from build123d import *

# Parameters (mm, degrees)
EXTRUDE1_DEPTH            = 32.5
SKETCH2_W                 = 70
SKETCH2_H                 = 1.7
CUT_EXTRUDE1_DEPTH        = 124.086646311
M5_CLEARANCE_HOLE1_D      = 5.5
M5X0_8_TAPPED_HOLE1_D     = 4.2
M5X0_8_TAPPED_HOLE1_DEPTH = 19.05
M5X0_8_TAPPED_HOLE1_TIP   = 1.2618073
F_5_0_5_DIAMETER_HOLE1_D  = 5
M8X1_25_TAPPED_HOLE1_D    = 6.8
F_6_0_6_DIAMETER_HOLE1_D  = 6


with BuildPart() as part:
    # Sketch1 → Extrude1 (new, symmetric)
    with BuildSketch(Plane.XY):
        with BuildLine():
            Line((0, 0), (98, 0))
            Line((98, 0), (98, 12.7))
            Line((98, 12.7), (25.4, 12.7))
            ThreePointArc((25.4, 12.7), (16.419743879, 16.419743879), (12.7, 25.4))
            Line((12.7, 25.4), (12.7, 36.35))
            Line((12.7, 36.35), (0, 36.35))
            Line((0, 36.35), (0, 0))
        make_face()
    extrude(amount=EXTRUDE1_DEPTH, both=True)

    # Sketch2 → Cut-Extrude1 (cut, through all)
    with BuildSketch(Plane(origin=(0, 0, -32.5), x_dir=(-1, 0, 0), z_dir=(0, 0, -1))):
        with Locations((-63, 11.85)):
            Rectangle(SKETCH2_W, SKETCH2_H)
    extrude(amount=-CUT_EXTRUDE1_DEPTH, mode=Mode.SUBTRACT)

    # M5 Clearance Hole1 (through all)
    with Locations(Plane.XZ):
        with Locations((53.7, 15), (91.7, 15), (91.7, -15), (53.7, -15)):
            Hole(M5_CLEARANCE_HOLE1_D / 2)

    # M5x0.8 Tapped Hole1
    with Locations(Plane(origin=(0, 36.35, 0), x_dir=(-1, 0, 0), z_dir=(0, 1, 0))):
        with Locations((-6.35, 22.5), (-6.35, -22.5)):
            Hole(M5X0_8_TAPPED_HOLE1_D / 2, depth=M5X0_8_TAPPED_HOLE1_DEPTH)
            with Locations((0, 0, -(M5X0_8_TAPPED_HOLE1_DEPTH + M5X0_8_TAPPED_HOLE1_TIP / 2))):  # 118° drill point
                Cone(0, M5X0_8_TAPPED_HOLE1_D / 2, M5X0_8_TAPPED_HOLE1_TIP, mode=Mode.SUBTRACT)

    # Ø5.0 (5) Diameter Hole1 (through all)
    with Locations(Plane.XZ):
        with Locations((46.70001183, 12), (46.70001183, -12)):
            Hole(F_5_0_5_DIAMETER_HOLE1_D / 2)

    # M8x1.25 Tapped Hole1 (through all)
    with Locations(Plane.XZ):
        with Locations((72.7, -15), (72.7, 15)):
            Hole(M8X1_25_TAPPED_HOLE1_D / 2)

    # Ø6.0 (6) Diameter Hole1 (through all)
    with Locations(Plane.XZ):
        with Locations((64.7, 0), (80.7, 0)):
            Hole(F_6_0_6_DIAMETER_HOLE1_D / 2)


solid = part.part
Read the model definition and answer for the solid it produces. Units are mm, in the model's axes. A direction names the side the tool comes from. Round coordinates to 2 decimals unless told otherwise and drop trailing zeros. Order: outer loops, then holes, each group sorted by start corner. A loop starts at its lowest first (then second) coordinate and runs counter-clockwise, first axis right, second up. Notation, with made-up numbers: (59.25, 41.25) - (113.25, 41.25) arc R17 ccw to (113.25, 48.25) - close; hole circle Ø1 at (58, 72). An arc over 180 degrees is marked (long way). Use one line per item in the form item = value. Start each with the question number.
(1) The part is cut by section B-B (y = 8.5). Count the separate pieces of the cut face and the enclosed holes in it, then the cut area to 3 significant figures.
(2) The part is cut by section D-D (x = 91.7). Give the vertices of the cut face in (y, z), then the cut area to 3 significant figures.
(3) The part is cut by section C-C (y = 29). Give the vertices of the cut face in (x, z), then the cut area to 3 significant figures.
(4) The part is cut by section A-A (x = 72.7). Give the vertices of the cut face in (y, z).
(5) For faces 5 (the face through (37, 10, -32.5)), 6 (the face through (63, 11, -8)), 7 (the face through (7.48, 26.69, -20.73)), determine the directions among +Z, -Z, +X, -X, +Y, -Y from which every point of the face is accessible in a straight line to the end or side of a thin tool.
(6) Flat-ended cylindrical pins translate along their axes: pin 1 Ø12 at (y, z) = (24, -18) entering from +X; pin 2 Ø3.5 at (y, z) = (32, -1.5) entering from +X; pin 3 Ø8 at (x, z) = (46.7, -12) entering from +Y; pin 4 Ø4.5 at (x, z) = (53.7, 15) entering from +Y. Find the tip coordinate at first contact, or state that the pin passes through.
(7) Determine the mould class of faces 1 (the face through (89.08, 5.58, -14.17)), 2 (the face through (98, 5, 0)), 3 (the face through (48, 0, 0)), 4 (the face through (51.08, 5.58, -14.17)) for opening direction X: +X half, -X half, draft (parallel to the pull), parting line (faces both ways), or undercut.
(8) Find the intervals of material crossed by line 1 along Z through (x, y) = (53.7, 7); line 2 along X through (y, z) = (30.5, -22.5); line 3 along X through (y, z) = (7.5, -13), in increasing order. Write a range as from..to.
Checked values:
q1.separate_pieces = 1
q1.enclosed_holes = 10
q1.area = 6,110 mm^2
q2.outline = (0, -32.5) - (11, -32.5) - (11, -17.75) - (0, -17.75) - close; (0, -12.25) - (11, -12.25) - (11, 12.25) - (0, 12.25) - close; (0, 17.75) - (11, 17.75) - (11, 32.5) - (0, 32.5) - close
q2.area = 594 mm^2
q3.outline = (0, -32.5) - (12.7, -32.5) - (12.7, 32.5) - (0, 32.5) - close; hole circle Ø4.2 at (6.35, -22.5); hole circle Ø4.2 at (6.35, 22.5)
q3.area = 798 mm^2
q4.outline = (0, -32.5) - (11, -32.5) - (11, -18.4) - (0, -18.4) - close; (0, -11.6) - (11, -11.6) - (11, 11.6) - (0, 11.6) - close; (0, 18.4) - (11, 18.4) - (11, 32.5) - (0, 32.5) - close
q5.face_5 = -Z, +X, -X, +Y, -Y
q5.face_6 = +Z, -Z, +X, +Y
q5.face_7 = +Y
q6.pin_1 = 15.08
q6.pin_2 = 12.7
q6.pin_3 = 11
q6.pin_4 = through
q7.face_1 = undercut
q7.face_2 = +X half
q7.face_3 = draft
q7.face_4 = undercut
q8.line_1 = -32.5..-17.75, -12.25..12.25, 17.75..32.5
q8.line_2 = 0..4.25, 8.45..12.7
q8.line_3 = 0..44.41, 48.99..51.81, 55.59..69.95, 75.45..89.81, 93.59..98
